Design review of the part built by this model. Coordinates are the model's own, in mm. A direction names the side the tool comes from. Give positions to 0.01 mm unless a question says otherwise; leave off trailing zeros. Loops run counter-clockwise (first coordinate to the right, second up) from the corner with the lowest first, then second, coordinate; pieces in that order, holes last. Notation, with made-up numbers: (89, 61.5) -> (146, 61.5) arc R17 ccw to (146, 85.5) -> close; hole circle Ø10 at (22, -9.75). An arc over 180 degrees is marked (long way). Use a Markdown table: item, result. Add a question column.
1. Add section A-A (y = -12). State the section outline as (x, z) points, and give its area (3 significant figures).
2. Add section C-C (x = 34.5). State the section outline as (y, z) points, and give its area (3 significant figures).
3. Add section B-B (z = -2). State the section outline as (x, y) points, and give its area (3 significant figures).
4. To check wall thickness, follow line 1 (X direction, y = -7, z = -2.75); line 2 (X direction, y = -31.4, z = 1.7); line 3 (X direction, y = 32, z = -1). State the ranges of each line that lie inside material, in increasing order.
5. Draft analysis for pull direction Y (two halves, no side actions). For faces 4 (the flat face through (-47.501, -33, 0)), 5 (the flat face through (36.499, -18, 1)), state which applies: pulls with the +Y half, pulls with the -Y half, needs draft (parallel to the pull), parting line crosses it, or undercut.
6. For pin 1 Ø1.5 at (y, z) = (-15.5, 1.5) entering from -X; pin 2 Ø2.5 at (y, z) = (1.5, -1) entering from -X; pin 3 Ø1.8 at (y, z) = (-2, -0.5) entering from +X; pin 4 Ø6 at (x, z) = (-2.5, -5) entering from +Y, all flat-tipped, find the tip position at first contact; note any pin that passes through.
7. For faces 1 (the flat face through (38, 7, 0)), 2 (the flat face through (-39.501, 0, 0)), 3 (the flat face through (-40, 28.5, 1)), list the 3-axis set-ups (+Z, -Z, +X, -X, +Y, -Y) from which the entire face can be reached by the end or side of a thin tool; tool diameter is ignored.
Autodesk Inventor part; units mm, degrees
ref_plane "Plano de trabajo3" through (-33.5, 29.3, -8) normal (0, 0, -1) x (0, 1, 0)
ref_plane "YZ Plane" through (0, 0, 0) normal (1, 0, 0) x (0, 1, 0)
ref_plane "XZ Plane" through (0, 0, 0) normal (0, 1, 0) x (-1, 0, 0)
sketch "Boceto1" plane through (0, 0, 0) normal (0, 0, 1) x (1, 0, 0)
  line L0 (-33.5009, -14) -> (-33.5009, 14)
  line L1 (-36.5009, -14) -> (-33.5009, -14)
  line L2 (-33.5009, 14) -> (-36.5009, 14)
  line L3 (-36.5009, 14) -> (-36.5009, -14)
  line L4 (36.4991, -36.5) -> (36.4991, 36.5)
  line L5 (-36.5009, -36.5) -> (36.4991, -36.5)
  line L6 (-36.5009, 36.5) -> (-36.5009, -36.5)
  line L7 (36.4991, 36.5) -> (-36.5009, 36.5)
  point P0 (0, 0)
extrude "Extrusión1" add sketch "Boceto1" along normal blind 3
sketch "Boceto2" plane through (0, 0, 3) normal (0, 0, 1) x (1, 0, 0)
  line L0 (36.5, 36.5) -> (-36.5, 36.5)
  line L1 (-36.5, 36.5) -> (-36.5, -36.5)
  line L2 (-36.5, -36.5) -> (36.5, -36.5)
  line L3 (36.5, -36.5) -> (36.5, 36.5)
  circle A0 centre (-31.4009, 31.4) radius 2.1
  circle A1 centre (-31.4009, -31.4) radius 2.1
  circle A2 centre (31.3991, -31.4) radius 2.1
  circle A3 centre (31.3991, 31.4) radius 2.1
  point P0 (0, 0)
hole "Agujero1" at (-31.4009, 31.4, 3) at (-31.4009, -31.4, 3) at (31.3991, -31.4, 3) at (31.3991, 31.4, 3) direction (0, 0, -1) diameter 3.2 depth 5
sketch "Boceto4" plane through (-36.5009, -36.5, 0) normal (-1, 0, 0) x (0, 0, 1)
  line L0 (0, 73) -> (0, 0)
  line L1 (0, 0) -> (3, 0)
  line L2 (3, 73) -> (3, 0)
  line L3 (0, 73) -> (3, 73)
  line L4 (3, 73) -> (0, 73)
  line L5 (0, 73) -> (0, 65)
  line L6 (0, 65) -> (3, 65)
  line L7 (3, 65) -> (3, 73)
  point P0 (0, 36.5)
  dimension "d9" = 8
extrude "Extrusión2" add sketch "Boceto4" along normal blind 8 contours L3 L2 L6 L0
sketch "Boceto5" plane through (-44.5009, -36.5, 0) normal (-1, 0, 0) x (0, 0, 1)
  line L0 (3, 65) -> (3, 73)
  line L1 (3, 73) -> (0, 73)
  line L2 (0, 73) -> (0, 65)
  line L3 (0, 65) -> (3, 65)
  line L4 (0, 73) -> (3, 65)
  circle A0 centre (1.5, 69) radius 6
  line L5 (0, 62) -> (3, 62)
  line L6 (3, 62) -> (3, 76)
  line L7 (3, 76) -> (0, 76)
  line L8 (0, 76) -> (0, 62)
  line L9 (0, 62) -> (3, 76) construction
  line L10 (3, 62) -> (0, 76) construction
  point P0 (0, 36.5)
  point P1 (3, 74.8095)
  point P2 (3, 63.1905)
  dimension "d12" = 12
extrude "Extrusión3" add sketch "Boceto5" along normal blind 3 contours L4 L1 L0 | L6 A0 L8 L3 | L3 L2 L4 | L1 L8 A0 L6 | L8 A0 L2
ref_plane "Plano de trabajo1" through (36.4991, 0, 3) normal (0, 1, 0) x (1, 0, 0)
ref_plane "Plano de trabajo2" through (-0.0009, -36.5, 0) normal (-1, 0, 0) x (0, 0, 1)
mirror "Simetría1" about plane through (36.4991, 0, 3) normal (0, 1, 0) of "Extrusión3", "Extrusión2"
mirror "Simetría2" about plane through (-0.0009, -36.5, 0) normal (-1, 0, 0) of "Extrusión3", "Extrusión2", "Simetría1"
sketch "Boceto6" plane through (36.4991, -28.5, 0) normal (1, 0, 0) x (0, 0, -1)
  line L0 (0, 14.5) -> (75, 14.5)
  arc A0 (75, 7) -> (78, 10) centre (75, 10) ccw
  line L1 (75, 7) -> (0, 7)
  line L2 (0, -8) -> (0, 7)
  line L3 (81, -8) -> (0, -8)
  line L4 (81, -8) -> (81, 65)
  line L5 (81, 65) -> (0, 65)
  line L6 (0, 50) -> (0, 65)
  line L7 (0, 50) -> (75, 50)
  arc A1 (75, 42.5) -> (78, 45.5) centre (75, 45.5) ccw
  line L8 (75, 42.5) -> (0, 42.5)
  line L9 (0, 14.5) -> (0, 42.5)
  line L10 (0, 42.5) -> (0, 14.5)
  line L11 (-3, 0) -> (0, 0)
  line L12 (0, 0) -> (0, 57)
  line L13 (0, 57) -> (-3, 57)
  line L14 (-3, 0) -> (-3, 57)
  line L15 (3, 35.5) -> (-3, 35.5)
  line L16 (-3, 35.5) -> (-3, 20.5)
  line L17 (-3, 20.5) -> (3, 20.5)
  line L18 (3, 20.5) -> (3, 35.5)
  line L19 (3, 35.5) -> (-3, 20.5) construction
  line L20 (-3, 35.5) -> (3, 20.5) construction
  arc A2 (78, 11.5) -> (75, 14.5) centre (75, 11.5) ccw
  line L21 (78, 11.5) -> (78, 10)
  arc A3 (78, 47) -> (75, 50) centre (75, 47) ccw
  line L22 (78, 47) -> (78, 45.5)
  point P0 (0, 28.5)
  point P1 (0, 28)
  dimension "d15" = 6
  dimension "d16" = 15
extrude "Extrusión4" add sketch "Boceto6" along normal blind 3 contours L17 L14 L15 L9 | L9 L15 L18 L17
mirror "Simetría3" about plane through (-0.0009, -36.5, 0) normal (-1, 0, 0) of "Extrusión4"
sketch "Boceto7" plane through (0, 0, 0) normal (0, 0, -1) x (-1, 0, 0)
  line L0 (-31.9991, -16) -> (-31.9991, 16)
  arc A0 (-24.3245, -32) -> (-31.9991, -24.3254) centre (-31.3991, -31.4) ccw
  arc A1 (-31.9991, 24.3254) -> (-24.3245, 32) centre (-31.3991, 31.4) ccw
  arc A2 (33.5009, -26.7524) -> (26.7533, -33.5) centre (31.4009, -31.4) ccw
  line L1 (33.5009, 17) -> (33.5009, -17)
  arc A3 (-26.7524, -33.5) -> (-33.5, -26.7524) centre (-31.4, -31.4) ccw
  arc A4 (-33.5, 26.7524) -> (-26.7524, 33.5) centre (-31.4, 31.4) ccw
  arc A5 (26.7524, 33.5) -> (33.5, 26.7524) centre (31.4, 31.4) ccw
  line L2 (33.5, -26.7524) -> (33.5, 26.7524)
  circle A6 centre (31.4, -31.4) radius 5.1004
  arc A7 (33.7068, -26.2968) -> (26.2977, -33.7059) centre (31.4009, -31.4) ccw
  line L3 (33, -26.7524) -> (33, 26.0334)
  arc A8 (26.2968, 33.7059) -> (33, 26.0334) centre (31.4, 31.4) ccw
  line L4 (-33.5, -26.7524) -> (-33.5, 26.7524)
  arc A9 (-33, 26.0334) -> (-26.2968, 33.7059) centre (-31.4, 31.4) ccw
  line L5 (-33, 26.0334) -> (-33, -26.0334)
  arc A10 (-26.2968, -33.7059) -> (-33, -26.0334) centre (-31.4, -31.4) ccw
  line L6 (-25.8, -42) -> (-25.8, 78)
  line L7 (25.8, -39) -> (25.8, 51)
  point P0 (0, 0)
  point P1 (-25.8, -31.4)
  point P2 (-25.8, 31.4)
  point P3 (25.8, 31.4)
  point P4 (25.8, -31.4)
  point P5 (33, -26.0331)
  dimension "d29" = 0.5
  dimension "d30" = 0.5
  dimension "d31" = 0.5
ref_plane "Plano de trabajo3" through (-33.5, 29.3, -8) normal (0, 0, -1) x (0, 1, 0)
extrude "Extrusión5" add sketch "Boceto7" along normal up to surface (8 mm away) contours A9 L6 A10 L5
properties part number "Tapa dispensador"
Taken from the geometry:
| question | item | result |
|---|---|---|
| 1 | outline | (-36.5, 0) -> (25.8, 0) -> (25.8, -8) -> (33, -8) -> (33, 0) -> (36.5, 0) -> (36.5, 3) -> (-36.5, 3) -> close |
| 1 | area | 277 mm^2 |
| 2 | outline | (-36.5, 0) -> (36.5, 0) -> (36.5, 3) -> (-36.5, 3) -> close |
| 2 | area | 219 mm^2 |
| 3 | outline | (-47.5, -37.37) -> (-44.5, -37.37) -> (-44.5, -27.63) -> (-47.5, -27.63) -> close; (-47.5, 27.63) -> (-44.5, 27.63) -> (-44.5, 37.37) -> (-47.5, 37.37) -> close; (-39.5, -8) -> (-36.5, -8) -> (-36.5, 7) -> (-39.5, 7) -> close; (25.8, -31.4) arc R5.6 cw to (33, -26.03) -> (33, 26.03) arc R5.6 cw to (25.8, 31.39) -> close; (36.5, -8) -> (39.5, -8) -> (39.5, 7) -> (36.5, 7) -> close; (44.5, -37.37) -> (47.5, -37.37) -> (47.5, -27.63) -> (44.5, -27.63) -> close; (44.5, 27.63) -> (47.5, 27.63) -> (47.5, 37.37) -> (44.5, 37.37) -> close |
| 3 | area | 592 mm^2 |
| 4 | line 1 | x = -39.5 to -36.5, 25.8 to 33, 36.5 to 39.5 |
| 4 | line 2 | x = -47.5 to -33, -29.8 to 29.8, 33 to 47.5 |
| 4 | line 3 | x = -47.5 to -44.5, 44.5 to 47.5 |
| 5 | face 4 | needs draft |
| 5 | face 5 | undercut |
| 6 | pin 1 | stops at x = -36.5 |
| 6 | pin 2 | stops at x = -39.5 |
| 6 | pin 3 | stops at x = 39.5 |
| 6 | pin 4 | passes through |
| 7 | face 1 | +Z, -Z, +X |
| 7 | face 2 | +Z, -Z, -X |
| 7 | face 3 | +Z, -Z |
